Answer from the drawing. Dimensions are ordinates in mm from the lowest x, y and z of the part. A direction names the side the tool comes from. Round coordinates to 2 decimals unless told otherwise and drop trailing zeros. Loops run counter-clockwise (first coordinate to the right, second up) from the corner with the lowest first, then second, coordinate; pieces in that order, holes last. Notation, with made-up numbers: (-7.75, 11.5) - (17.25, 11.5) arc R11 cw to (17.25, 25.5) - close; hole circle Ø6 at (11.25, 32.5). An arc over 180 degrees is marked (long way). Answer as CSV lines item,"result".
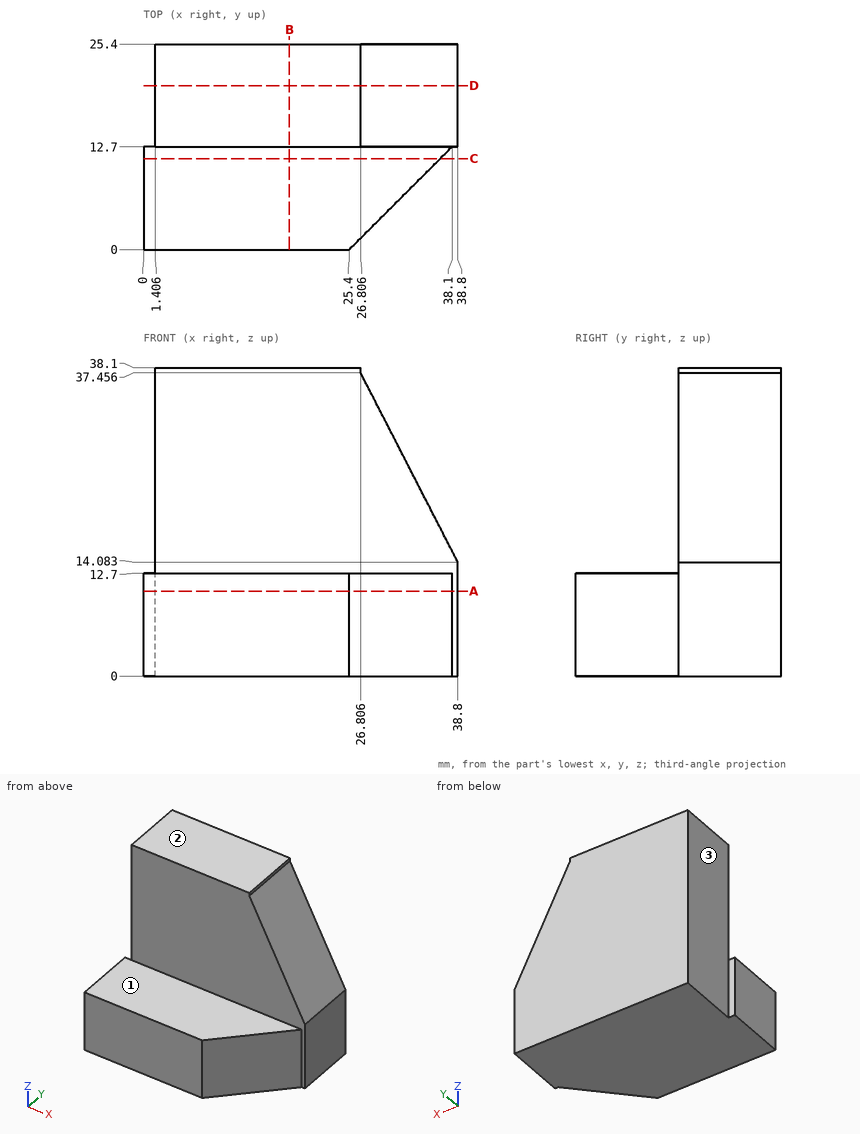
1) A cutting plane is placed at A-A, the plane z = 10.5. Determine the outline of the cut face in (x, y), plus the area to 3 significant figures.
Entries:
outline,"(0, 0) - (25.4, 0) - (38.1, 12.7) - (38.8, 12.7) - (38.8, 25.4) - (1.41, 25.4) - (1.41, 12.7) - (0, 12.7) - close"
area,"878 mm^2"
2) A cutting plane is placed at C-C, the plane y = 11.25. Determine the outline of the cut face in (x, z).
Entries:
outline,"(0, 0) - (36.65, 0) - (36.65, 12.7) - (0, 12.7) - close"
3) Find the intervals of material crossed by line 1 (Z direction, x = 24.5, y = 1.5); line 2 (Y direction, x = 14, z = 26); line 3 (X direction, y = 20.25, z = 11), in increasing order.
Entries:
line 1,"z = 0 to 12.7"
line 2,"y = 12.7 to 25.4"
line 3,"x = 1.41 to 38.8"
4) A cutting plane is placed at B-B, the plane x = 18. Determine the outline of the cut face in (y, z).
Entries:
outline,"(0, 0) - (25.4, 0) - (25.4, 38.1) - (12.7, 38.1) - (12.7, 12.7) - (0, 12.7) - close"
5) A tool of negligible diameter and unlimited length cuts with its end or side. For the marked faces 1, 2 and 3, from which of +Z, -Z, +X, -X, +Y, -Y can it reach the whole face along a straight path? Write none if from no direction.
Entries:
face 1,"+Z, +X, -X, -Y"
face 2,"+Z, +X, -X, +Y, -Y"
face 3,"+Z, -Z, -X, +Y"
6) A cutting plane is placed at D-D, the plane y = 20.25. Determine the outline of the cut face in (x, z) (1 decimal), plus the area to 3 significant figures.
Entries:
outline,"(1.4, 0) - (38.8, 0) - (38.8, 14.1) - (26.8, 37.5) - (26.8, 38.1) - (1.4, 38.1) - close"
area,"1,280 mm^2"
7) Each of these flat-tipped pins is pushed along its axis until it touches: P1, Ø4, axis at y = 20.5, z = 24.5, coming from the -X side; P2, Ø5, axis at x = 6, z = 11.5, coming from the -Y side; P3, Ø14, axis at x = 14, y = 3.5, coming from the +Z side; P4, Ø8, axis at y = 6, z = 27, coming from the +X side. Where does it stop, or does it pass through?
Entries:
P1,"stops at x = 1.41"
P2,"stops at y = 0"
P3,"stops at z = 12.7"
P4,"passes through"
